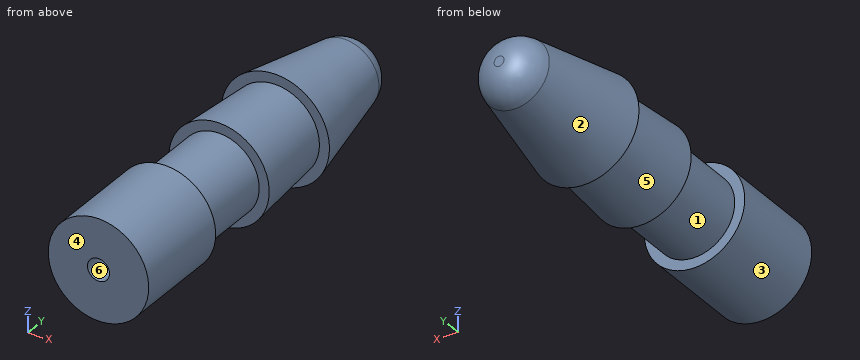
Autodesk Fusion 360 part; units mm, degrees
sketch "Sketch1" plane through (0, 0, 0) normal (1, 0, 0) x (0, 1, 0)
  line L0 (0, 0) -> (0, 12.5)
  line L1 (0, 12.5) -> (25, 12.5)
  line L2 (25, 12.5) -> (25, 10)
  line L3 (25, 10) -> (45, 10)
  line L4 (45, 10) -> (45, 12.5)
  line L5 (45, 12.5) -> (66, 12.5) construction
  line L6 (66, 12.5) -> (66, 11)
  line L7 (45, 12.5) -> (66, 11)
  line L8 (66, 12.5) -> (66, 13.5)
  line L9 (66, 13.5) -> (92, 13.5) construction
  line L10 (92, 13.5) -> (92, 8.5) construction
  line L11 (66, 13.5) -> (92, 8.5)
  line L12 (66, 13.5) -> (98, 13.5) construction
  line L13 (98, 13.5) -> (98, 0)
  arc A0 (98, 1.2362) -> (92, 8.5) centre (90.6031, 1.2362) ccw
  line L14 (98, 0) -> (0, 0)
  dimension "d1" = 12.5
  dimension "d2" = 25
  dimension "d4" = 20
  dimension "d6" = 21
  dimension "d9" = 26
  dimension "d10" = 5
  dimension "d11" = 13.5
  dimension "d12" = 12.5
  dimension "d13" = 10
  dimension "d14" = 11
  dimension "d15" = 32
  dimension "d16" = 7.3969
revolve "Revolve1" add sketch "Sketch1" angle 360 about axis through (0, 98, 0) along (0, -1, 0)
sketch "Sketch3" plane through (0, 0, 0) normal (0, -1, 0) x (1, 0, 0)
  circle A0 centre (0, 0) radius 12.5
  circle A1 centre (0, 0) radius 2.75
  dimension "d26" = 5.5
extrude "Extrude2" cut sketch "Sketch3" against normal blind 12.5 contours A1
equation "d1 = 25 mm / 2"
Input: part model. Units: mm. Frame: model coordinates. Face numbers are marked on the shaded views. A direction names the side the tool comes from. Round coordinates to 2 decimals unless told otherwise and drop trailing zeros. Order: outer loops, then holes, each group sorted by start corner. A loop starts at its lowest first (then second) coordinate and runs counter-clockwise, first axis right, second up. Notation, with made-up numbers: (35.5, 39.25) - (42.5, 39.25) arc R22 cw to (42.5, 63.25) - close; hole circle Ø7 at (9.25, 1.5). An arc over 180 degrees is marked (long way). One line per question, with ' | ' between items. Start each with the question number.
1) Cut plane A-A, the plane y = 15. Return the cut outline in (x, z), then the cut area to 3 significant figures.
2) Pull-direction query (Z, two-part tool) for the marked faces 4, 5 and 6; classes: +Z half, -Z half, draft (parallel to the pull), parting line (faces both ways), or undercut.
3) Ray query, probe 1 along Z at (x, y) = (0, 3.75); probe 2 along Y at (x, z) = (1, 1); probe 3 along Z at (x, y) = (3.5, 57). Return the intervals inside material, ascending.
4) Set-up query: the marked faces 1, 2 and 3. Return all of +Z, -Z, +X, -X, +Y, -Y with unobstructed straight access to the full face (end or side cutting, diameter ignored); none if empty.
5) Cut plane B-B, the plane y = 49. Return the cut outline in (x, z), then the cut area to 3 significant figures.
6) Contact query for flat-ended pins moving along their axis: P1, Ø13.5, axis at x = -2, z = 5.5, coming from the -Y side; P2, Ø8, axis at x = 9, z = 3, coming from the +Y side; P3, Ø8, axis at x = 1.5, y = 70.5, coming from the +Z side; P4, Ø2, axis at x = -3.5, z = 4.5, coming from the +Y side. Output: stop coordinate, or through.
Worked out:
1) outline: circle Ø25 at (0, 0) | area: 491 mm^2
2) face 4: draft | face 5: parting line | face 6: undercut
3) probe 1: z = -12.5 to -2.75, 2.75 to 12.5 | probe 2: y = 12.5 to 98 | probe 3: z = -11.1 to 11.1
4) face 1: none | face 2: +Y | face 3: -Y
5) outline: circle Ø24.43 at (0, 0) | area: 469 mm^2
6) P1: stops at y = 0 | P2: stops at y = 96.66 | P3: stops at z = 13.37 | P4: stops at y = 97.14
